Source: CAD feature listing. Evaluate the final solid. Frame: model axes, mm. A direction names the side the tool comes from. Coordinates: 2 decimals unless noted, no trailing zeros. Order: outer loops, then holes, each group sorted by start corner. A loop starts at its lowest first (then second) coordinate and runs counter-clockwise, first axis right, second up. Notation, with made-up numbers: (-16, 78) -> (8, 78) arc R16 ccw to (8, 109) -> close; hole circle Ø6 at (1, 11). An arc over 180 degrees is marked (long way). Write item = value, one per line. Start each with the question number.
Item 1: Set-up query: faces 1 (the flat face through (3.9, -6.23, 0.99)), 2 (the flat face through (-12, 23, 1.2)), 3 (the flat face through (9, -6.512, 1)). Return all of +Z, -Z, +X, -X, +Y, -Y with unobstructed straight access to the full face (end or side cutting, diameter ignored); none if empty.
Item 2: Contact query for flat-ended pins moving along their axis: pin 1 (10 mm diameter, centred on x = -13, y = 6.5, fed in from +Z); pin 2 (8 mm diameter, centred on x = -5.5, y = 23, fed in from +Z). Output: stop coordinate, or through.
Item 3: Section query A-A (z = 0.55). Output: boundary loops of the cut face in (x, y) (3 decimals), then the cut area to 3 significant figures.
Item 4: Ray query, line 1 along Y through (x, z) = (0, 1.55) (3 decimals); line 2 along Z through (x, y) = (-9.5, 15); line 3 along Y through (x, z) = (0, 0.55) (3 decimals). Return the intervals inside material, ascending. Write a range as [from, to].
Item 5: Mould query, pull axis Y, two halves, no side actions, for faces 4 (the flat face through (7, -10.212, 1)), 5 (the flat face through (1.2, -3.3, 2)), 6 (the flat face through (4.387, -5.704, 0.986)), 7 (the flat face through (-23.317, 38.608, 0.592)). Classes: released by +Y, released by -Y, zero draft, split by the parting line, or undercut.
Item 6: Section query B-B (y = 6). Output: boundary loops of the cut face in (x, z), then the cut area to 3 significant figures.
Item 7: Section query D-D (y = 20.5). Output: boundary loops of the cut face in (x, z).
Item 8: Section query C-C (x = -20). Output: boundary loops of the cut face in (y, z).
```python
from build123d import *

# Parameters (mm, degrees)
SKETCH1_R           = 3.175
BOSS_EXTRUDE1_DEPTH = 1.2
SKETCH2_R           = 3.175
BOSS_EXTRUDE2_DEPTH = 0.8


with BuildPart() as part:
    # Sketch1 → Boss-Extrude1 (new body)
    with BuildSketch(Plane.XY):
        Polygon((-0.387763394, -10.212000445), (-7.602233748, 0.091331011), (-5.023989087, 7.175), (-25.810939636, 36.861841993), (-20.752675762, 40.403676487), (12.098034886, -6.512000445), (4.952577098, -6.512000445), (3.805424226, -4.873696357), (3.232017795, -5.275199862), (4.588180163, -7.212000445), (12.588180163, -7.212000445), (14.688802778, -10.212000445), align=None)
        Circle(SKETCH1_R, mode=Mode.SUBTRACT)
    extrude(amount=BOSS_EXTRUDE1_DEPTH)

    # Sketch2 → Boss-Extrude2 (add)
    with BuildSketch(Plane.XY.offset(1.2)):
        Polygon((-5.023989087, 7.175), (2.514293999, 7.175), (12.098034886, -6.512000445), (4.952577098, -6.512000445), (3.805424226, -4.873696357), (3.232017795, -5.275199862), (4.588180163, -7.212000445), (12.588180163, -7.212000445), (14.688802778, -10.212000445), (-0.387763394, -10.212000445), (-7.602233748, 0.091331011), align=None)
        Circle(SKETCH2_R, mode=Mode.SUBTRACT)
    extrude(amount=BOSS_EXTRUDE2_DEPTH)


solid = part.part
```
Computed:
q1.face_1 = +Z, -Z
q1.face_2 = +Z, +X, -X, +Y
q1.face_3 = +Z, -Z, +X
q2.pin_1 = through
q2.pin_2 = 1.2
q3.outline = (-25.811, 36.862) -> (-5.024, 7.175) -> (-7.602, 0.091) -> (-0.388, -10.212) -> (14.689, -10.212) -> (12.588, -7.212) -> (4.588, -7.212) -> (3.232, -5.275) -> (3.805, -4.874) -> (4.953, -6.512) -> (12.098, -6.512) -> (-20.753, 40.404) -> close; hole circle Ø6.35 at (0, 0)
q3.area = 434 mm^2
q4.line_1 = [-10.212, -3.175], [3.175, 7.175]
q4.line_2 = [0, 1.2]
q4.line_3 = [-10.212, -3.175], [3.175, 10.766]
q5.face_4 = released by -Y
q5.face_5 = zero draft
q5.face_6 = undercut
q5.face_7 = released by +Y
q6.outline = (-5.45, 0) -> (3.34, 0) -> (3.34, 2) -> (-5.45, 2) -> close
q6.area = 17.6 mm^2
q7.outline = (-14.35, 0) -> (-6.82, 0) -> (-6.82, 1.2) -> (-14.35, 1.2) -> close
q8.outline = (28.56, 0) -> (39.33, 0) -> (39.33, 1.2) -> (28.56, 1.2) -> close
